The listing builds one solid part. Answer for the finished solid, in the listing's coordinates (mm). Face numbers are marked on the shaded views. A direction names the side the tool comes from. Round coordinates to 2 decimals unless told otherwise and drop trailing zeros. Loops run counter-clockwise (first coordinate to the right, second up) from the corner with the lowest first, then second, coordinate; pieces in that order, holes last. Notation, with made-up numbers: M 56.25,67.25 L 60.25,67.25 A26 cw 60.25,82.25 Z; hole C 76.5,42 d7. An arc over 180 degrees is marked long. Answer as a JSON object with one key per item and string values.
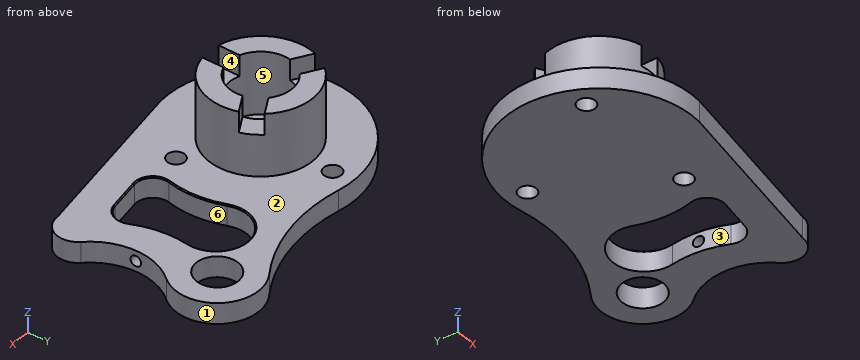
Autodesk Inventor part; units mm, degrees
ref_plane "Work Plane1" through (70.1484, 13.0405, 0) normal (-1, 0, 0) x (0, 0, 1)
ref_plane "YZ Plane" through (0, 0, 0) normal (1, 0, 0) x (0, 1, 0)
ref_plane "XZ Plane" through (0, 0, 0) normal (0, 1, 0) x (-1, 0, 0)
sketch "Sketch1" plane through (0, 0, 0) normal (0, 0, 1) x (1, 0, 0)
  arc A0 (93.3944, 27.2324) -> (66.8467, 56.6014) centre (78, 40) ccw
  circle A1 centre (78, 40) radius 10
  arc A2 (88.012, -30) -> (95.1215, -12.9797) centre (88, -20) ccw
  arc A3 (93.3944, 27.2324) -> (95.1215, -12.9797) centre (116.4861, 8.081) ccw
  arc A4 (70.653, 19.7601) -> (41.8659, 16.5) centre (55.8211, 22) ccw
  line L0 (5.1648, -44.7026) -> (88.012, -30)
  line L1 (53.0014, -19.9632) -> (68.5014, -17.2125)
  arc A5 (70.653, 19.7601) -> (74.3556, -5.958) centre (115.1484, 13.0405) ccw
  arc A6 (43.8143, -10.2619) -> (53.0014, -19.9632) centre (51.6035, -12.0863) ccw
  arc A7 (68.5014, -17.2125) -> (74.3556, -5.958) centre (67.1035, -9.3356) ccw
  arc A8 (8.0041, 44.2824) -> (66.8467, 56.6014) centre (22.2337, 123.0068) ccw
  arc A9 (43.8143, -10.2619) -> (41.8659, 16.5) centre (0, 0) ccw
  arc A10 (8.0041, 44.2824) -> (5.1648, -44.7026) centre (0, 0) ccw
  dimension "d1" = 40
  dimension "d2" = 20
  dimension "d3" = 40
  dimension "d4" = 78
  dimension "d5" = 20
  dimension "d6" = 20
  dimension "d7" = 88
  dimension "d8" = 60
  dimension "d10" = 30
  dimension "d11" = 22
  dimension "d19" = 16
  dimension "d22" = 15.5
  dimension "d23" = 90
  dimension "d24" = 160
  dimension "d25" = 45
  dimension "d26" = 123.0068
  dimension "d27" = 44.9174
  dimension "d28" = 8
  dimension "d29" = 8
  dimension "d31" = 45
  dimension "d32" = 31.3356
  dimension "d33" = 34.0863
  dimension "d34" = 13.0404
  dimension "d70" = 55.8211
extrude "Extrusion1" add sketch "Sketch1" along normal blind 10
sketch "Sketch2" plane through (0, 0, 10) normal (0, 0, 1) x (1, 0, 0)
  circle A0 centre (0, 0) radius 25
  circle A1 centre (0, 0) radius 15
  dimension "d37" = 50
  dimension "d38" = 30
extrude "Extrusion2" add sketch "Sketch2" along normal blind 30
sketch "Sketch3" plane through (0, 0, 40) normal (0, 0, 1) x (1, 0, 0)
  line L0 (-5, -12.5) -> (5, -12.5)
  line L1 (5, -12.5) -> (5, -27.5)
  line L2 (5, -27.5) -> (-5, -27.5)
  line L3 (-5, -27.5) -> (-5, -12.5)
  line L4 (-5, -12.5) -> (5, -27.5) construction
  line L5 (5, -12.5) -> (-5, -27.5) construction
  line L6 (13.3253, 1.9199) -> (8.3253, 10.5801)
  line L7 (26.3157, 9.4199) -> (13.3253, 1.9199)
  line L8 (8.3253, 10.5801) -> (21.3157, 18.0801)
  line L9 (21.3157, 18.0801) -> (26.3157, 9.4199)
  line L10 (-8.3253, 10.5801) -> (-13.3253, 1.9199)
  line L11 (-21.3157, 18.0801) -> (-8.3253, 10.5801)
  line L12 (-13.3253, 1.9199) -> (-26.3157, 9.4199)
  line L13 (-26.3157, 9.4199) -> (-21.3157, 18.0801)
  point P0 (0, 0)
  point P1 (0, -20)
  dimension "d41" = 20
  dimension "d42" = 10
  dimension "d43" = 15
  dimension "d44" = 12.5
  dimension "d47" = 360
extrude "Extrusion3" cut sketch "Sketch3" against normal blind 10
sketch "Sketch4" plane through (0, 0, 10) normal (0, 0, 1) x (1, 0, 0)
  point P0 (0, 0)
  point P1 (0, 35)
  dimension "d51" = 35
hole "Hole1" at (0, 35, 10) direction (0, 0, -1) diameter 8.376 end through all
ref_plane "Work Plane1" through (70.1484, 13.0405, 0) normal (-1, 0, 0) x (0, 0, 1)
sketch "Sketch5" plane through (70.1484, 13.0405, 0) normal (-1, 0, 0) x (0, 0, 1)
  circle A0 centre (5, -6.0202) radius 2.5
  line L0 (0, 14.192) -> (0, -26.0202)
  line L1 (0, -26.0202) -> (10, -26.0202)
  point P0 (0, -13.0405)
  dimension "d59" = 5
  dimension "d60" = 5
  dimension "d61" = 20
extrude "Extrusion4" cut sketch "Sketch5" against normal through all
pattern_circular "Circular Pattern1" count 3 over 360 about axis through (0, 0, 0) along (0, 0, 1) of "Hole1"
chamfer "Chamfer1" distance 0.5 angle 45 6 edges at (54.1332, 36.9047, 10) (70.6077, 6.628, 10) (74.2008, -13.0273, 10) (60.7514, -18.5878, 10) (45.7948, -17.5871, 10) (44.8812, 3.2676, 10)
properties part number "Curved disk example"
Item 1: Straight lines are drawn through the part: line 1 (Z direction, x = 81.5, y = 7); line 2 (Y direction, x = 0, z = 7); line 3 (X direction, y = 0, z = 28.75). For each, find the intervals that lie inside material, in ascending order.
Values follow:
{"line 1": "0 to 2.5, 7.5 to 10", "line 2": "-45 to 30.81, 39.19 to 45", "line 3": "-25 to -15, 15 to 25"}
Item 2: Which of the six approach directions +Z, -Z, +X, -X, +Y, -Y give full straight-line access (tool end or side, diameter ignored) to the marked faces 4, 5 and 6?
Values follow:
{"face 4": "+Z, -Y", "face 5": "+Z", "face 6": "+Z, -Z"}
Item 3: Determine the mould class of the marked faces 1, 2 and 3 for opening direction X: released by +X, released by -X, zero draft, split by the parting line, or undercut.
Values follow:
{"face 1": "split by the parting line", "face 2": "zero draft", "face 3": "undercut"}
Item 4: Flat-ended cylindrical pins translate along their axes: P1, Ø6, axis at x = 36.5, z = 11, coming from the -Y side; P2, Ø4, axis at x = 20, y = 9, coming from the +Z side; P3, Ø6.5, axis at x = -30.31, y = -17.5, coming from the +Z side; P4, Ø3, axis at y = -17.5, z = 36, coming from the -X side. Find the tip coordinate at first contact, or state that the pin passes through.
Values follow:
{"P1": "y = -39.64", "P2": "z = 30", "P3": "through", "P4": "x = -19.21"}
Item 5: The part is cut by section A-A (x = 78). Give the vertices of the cut face in (y, z).
Values follow:
{"outline": "M -31.78,0 L 30,0 L 30,10 L -31.78,10 Z; M 50,0 L 60,0 L 60,10 L 50,10 Z; hole C 7.02,5 d5"}
Item 6: The part is cut by section B-B (x = 0). Give the vertices of the cut face in (y, z).
Values follow:
{"outline": "M -45,0 L 30.81,0 L 30.81,10 L 25,10 L 25,40 L 15,40 L 15,10 L -15,10 L -15,30 L -25,30 L -25,10 L -45,10 Z; M 39.19,0 L 45,0 L 45,10 L 39.19,10 Z"}
Item 7: The part is cut by section C-C (z = 5). Give the vertices of the cut face in (x, y).
Values follow:
{"outline": "M 5.16,-44.7 L 88.01,-30 A10 ccw 95.12,-12.98 A30 cw 86.7,4.52 L 70.96,4.52 A45 ccw 74.36,-5.96 A8 cw 68.5,-17.21 L 53,-19.96 A8 cw 43.81,-10.26 A45 ccw 41.87,16.5 A15 cw long 70.65,19.76 A45 ccw 70.29,9.52 L 86.52,9.52 A30 cw 93.39,27.23 A20 ccw 66.85,56.6 A80 cw 8,44.28 A45 ccw long Z; hole C -30.31,-17.5 d8.38; hole C 0,35 d8.38; hole C 30.31,-17.5 d8.38; hole C 78,40 d20"}
Item 8: The part is cut by section D-D (z = 19.5). Give the vertices of the cut face in (x, y), then the cut area to 3 significant figures.
Values follow:
{"outline": "C 0,0 d50; hole C 0,0 d30", "area": "1,260 mm^2"}
